CAD build for the part. Positions are in the model's coordinates, mm. Face numbers are marked on the shaded views. A direction names the side the tool comes from. Coordinates: 2 decimals unless noted, no trailing zeros. Loops run counter-clockwise (first coordinate to the right, second up) from the corner with the lowest first, then second, coordinate; pieces in that order, holes last.
1) Saw through at B-B, the plane x = 1. Write the cut outline in (y, z), and give its area (3 significant figures).
2) Saw through at A-A, the plane y = 3. Write the cut outline in (x, z).
3) Wall check: line 1 along Y through (x, z) = (30, 6.75); line 2 along Y through (x, z) = (-13, 7); line 3 along X through (y, z) = (7, 4.5). Give the ranges that are in metal, low to high.
4) Which spindle directions (+Z, -Z, +X, -X, +Y, -Y) get a long thin tool onto all of the face, cutting with end or side? Do the marked faces 1 and 2. Say none if no direction does.
5) Saw through at C-C, the plane y = -29. Write the cut outline in (x, z), and give its area (3 significant figures).
6) Two-plate mould, pull along X, no slides. Class the marked faces 3 and 4: +X half, -X half, draft (parallel to the pull), parting line (faces both ways), or undercut.
7) Saw through at D-D, the plane x = -44. Write the cut outline in (y, z).
8) Pin check, flat tips, straight feed: pin 1 Ø2.5 at (x, z) = (-3.5, 6.5) entering from +Y; pin 2 Ø3.5 at (x, z) = (28.5, 6.5) entering from +Y; pin 3 Ø3 at (y, z) = (-9.5, 6) entering from +X. Stop position of each tip, or through.
```python
from build123d import *

# Parameters (mm, degrees)
F0_W     = 100
F0_H     = 100
F1_DEPTH = 4
F3_DEPTH = 4
F5_DEPTH = 3


with BuildPart() as f1:
    # F0 (on Top) → F1 (new body)
    with BuildSketch(Plane.XY):
        Rectangle(F0_W, F0_H)
    extrude(amount=F1_DEPTH)

    # F2 (on face) → F3 (join)
    with BuildSketch(Plane.XY.offset(4)):
        Polygon((35, -15), (35, 15), (15, 35), (0, 35), (-15, 35), (-35, 15), (-35, -15), (-15, -35), (0, -35), (15, -35), align=None)
    extrude(amount=F3_DEPTH)

    # F4 (on face) → F5 (cut)
    with BuildSketch(Plane.XY.offset(8)):
        with BuildLine():
            Line((15, 20), (-15, 20))
            ThreePointArc((-15, 20), (-18.535534, 18.535534), (-20, 15))
            Line((-20, 15), (-20, 6))
            Line((-20, 6), (-35, 6))
            Line((-35, 6), (-35, -6))
            Line((-35, -6), (-20, -6))
            Line((-20, -6), (-20, -15))
            ThreePointArc((-20, -15), (-18.535534, -18.535534), (-15, -20))
            Line((-15, -20), (15, -20))
            ThreePointArc((15, -20), (18.535534, -18.535534), (20, -15))
            Line((20, -15), (20, -6))
            Line((20, -6), (35, -6))
            Line((35, -6), (35, 6))
            Line((35, 6), (20, 6))
            Line((20, 6), (20, 15))
            ThreePointArc((20, 15), (18.535534, 18.535534), (15, 20))
        make_face()
    extrude(amount=-F5_DEPTH, mode=Mode.SUBTRACT)


solid = f1.part
```
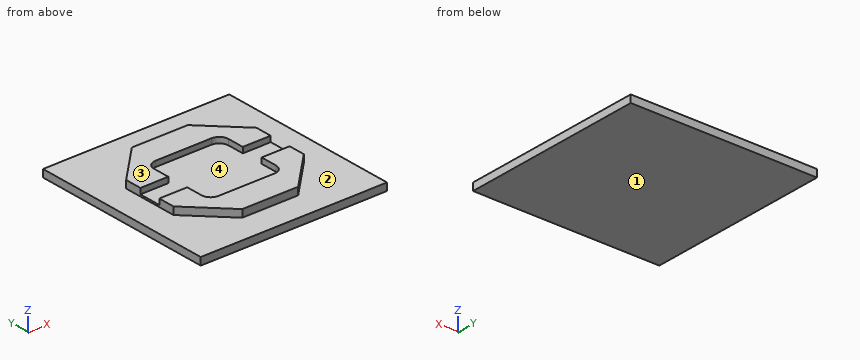
Data:
1. outline: (-50, 0) - (50, 0) - (50, 4) - (35, 4) - (35, 8) - (20, 8) - (20, 5) - (-20, 5) - (-20, 8) - (-35, 8) - (-35, 4) - (-50, 4) - close
1. area: 560 mm2
2. outline: (-50, 0) - (50, 0) - (50, 4) - (35, 4) - (35, 5) - (-35, 5) - (-35, 4) - (-50, 4) - close
3. line 1: y = -20 to -6, 6 to 20
3. line 2: y = -35 to -20, 20 to 35
3. line 3: x = -35 to 35
4. face 1: -Z, +X, -X, +Y, -Y
4. face 2: +Z
5. outline: (-50, 0) - (50, 0) - (50, 4) - (21, 4) - (21, 8) - (-21, 8) - (-21, 4) - (-50, 4) - close
5. area: 568 mm2
6. face 3: draft
6. face 4: undercut
7. outline: (-50, 0) - (50, 0) - (50, 4) - (-50, 4) - close
8. pin 1: stops at y = 35
8. pin 2: stops at y = 23.25
8. pin 3: stops at x = 35
